```python
from build123d import *

# Parameters (mm, degrees)
F0_R     = 6.35
F1_DEPTH = 127
F2_SIZE2 = 1.524
F2_SIZE  = 1.524
F3_R     = 2.38125
F4_DEPTH = 10.414
F5_SIZE2 = 0.508
F5_SIZE  = 0.508


with BuildPart() as f1:
    # F0 (on Right) → F1 (new body)
    with BuildSketch(Plane.YZ):
        Circle(F0_R)
    extrude(amount=F1_DEPTH)

    # F2
    f2_edges = [f1.edges().sort_by_distance(p)[0] for p in [
        (127, -6.35, 0),
    ]]
    chamfer(f2_edges, length=F2_SIZE, length2=F2_SIZE2)

    # F3 (on Right) → F4 (join)
    with BuildSketch(Plane.YZ):
        Circle(F3_R)
    extrude(amount=-F4_DEPTH)

    # F5
    f5_edges = [f1.edges().sort_by_distance(p)[0] for p in [
        (0, -6.35, 0),
        (-10.414, -2.38125, 0),
    ]]
    chamfer(f5_edges, length=F5_SIZE, length2=F5_SIZE2)


solid = f1.part
```
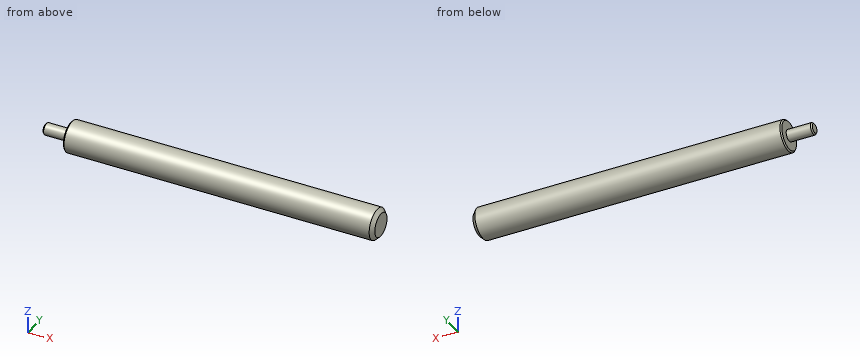
The model under review builds one solid part; all positions refer to its coordinate system, in mm. Coordinates: 2 decimals unless noted, no trailing zeros. Write each loop counter-clockwise with the first axis right and the second up, starting at its lowest first coordinate (ties: lowest second). Pieces come first, ordered by that corner, then holes. Notation, with made-up numbers: (-13, 77.5) -> (25, 77.5) arc R19 ccw to (25, 111.5) -> close; hole circle Ø7 at (-9, 60). An arc over 180 degrees is marked (long way). One line per item, written item: value. Start each with the question number.
Q1. Add section C-C, the plane x = 79. Give the boundary of the cut face in (y, z).
Q2. Clearance check with flat-ended pins moving along their axes: P1, Ø4, axis at x = 51, y = 2.5, coming from the +Z side; P2, Ø1, axis at y = -1.5, z = 3, coming from the -X side; P3, Ø3, axis at y = 3.5, z = 1, coming from the -X side. State where each tip first meets the part, or that it passes through.
Q3. Add section A-A, the plane y = 0. Give the boundary of the cut face in (x, z).
Q4. To check wall thickness, follow probe 1 along Z at (x, y) = (0.5, 0.5); probe 2 along X at (y, z) = (0.75, 3); probe 3 along Y at (x, z) = (26, -3.75). State the ranges of each line that lie inside material, in increasing order.
Response:
1. outline: circle Ø12.7 at (0, 0)
2. P1: z = 6.33
2. P2: x = 0
2. P3: x = -10.15
3. outline: (-10.41, -1.87) -> (-9.91, -2.38) -> (0, -2.38) -> (0, -5.84) -> (0.51, -6.35) -> (125.48, -6.35) -> (127, -4.83) -> (127, 4.83) -> (125.48, 6.35) -> (0.51, 6.35) -> (0, 5.84) -> (0, 2.38) -> (-9.91, 2.38) -> (-10.41, 1.87) -> close
4. probe 1: -6.32 to 6.32
4. probe 2: 0 to 127
4. probe 3: -5.12 to 5.12
